Read the model definition and answer for the solid it produces. Units are mm, in the model's axes. Round coordinates to 2 decimals unless told otherwise and drop trailing zeros. Loops run counter-clockwise (first coordinate to the right, second up) from the corner with the lowest first, then second, coordinate; pieces in that order, holes last. Notation, with made-up numbers: M -23.75,72 L -16.75,72 A30 ccw -16.75,101 Z; hole C 28.25,42 d11. An arc over 180 degrees is marked long. Answer as CSV lines item,"result".
Autodesk Inventor part; units mm, degrees
ref_plane "YZ Plane" through (0, 0, 0) normal (1, 0, 0) x (0, 1, 0)
ref_plane "XZ Plane" through (0, 0, 0) normal (0, 1, 0) x (-1, 0, 0)
ref_plane "XY Plane" through (0, 0, 0) normal (0, 0, 1) x (1, 0, 0)
sketch "Sketch1" plane through (0, 0, 0) normal (0, 0, 1) x (1, 0, 0)
  circle A0 centre (0, 0) radius 15.875
  arc A1 (-3.0359, 9.528) -> (-6.5275, 7.5757) centre (0, 0) ccw
  line L0 (0, 0) -> (-5, 8.6603) construction
  line L1 (0, 0) -> (-10.16, 0) construction
  line L2 (-2.058, 7.8342) -> (-3.0359, 9.528)
  line L3 (-5.5564, 5.8937) -> (-6.5275, 7.5757)
  arc A2 (-2.058, 7.8342) -> (-5.5564, 5.8937) centre (0, 0) ccw
  circle A3 centre (0, 0) radius 8.1
  arc A4 (6.7336, 7.3932) -> (3.297, 9.4409) centre (0, 0) ccw
  line L4 (5.7556, 5.6994) -> (6.7336, 7.3932)
  line L5 (2.3259, 7.7589) -> (3.297, 9.4409)
  arc A5 (9.7695, -2.1348) -> (9.8245, 1.8652) centre (0, 0) ccw
  line L6 (7.8136, -2.1348) -> (9.7695, -2.1348)
  line L7 (7.8823, 1.8652) -> (9.8245, 1.8652)
  arc A6 (3.0359, -9.528) -> (6.5275, -7.5757) centre (0, 0) ccw
  line L8 (2.058, -7.8342) -> (3.0359, -9.528)
  line L9 (5.5564, -5.8937) -> (6.5275, -7.5757)
  arc A7 (-6.7336, -7.3932) -> (-3.297, -9.4409) centre (0, 0) ccw
  line L10 (-5.7556, -5.6994) -> (-6.7336, -7.3932)
  line L11 (-2.3259, -7.7589) -> (-3.297, -9.4409)
  arc A8 (-9.7695, 2.1348) -> (-9.8245, -1.8652) centre (0, 0) ccw
  line L12 (-7.8136, 2.1348) -> (-9.7695, 2.1348)
  line L13 (-7.8823, -1.8652) -> (-9.8245, -1.8652)
  point P0 (5, 8.6603)
  point P1 (10, 0)
  point P2 (5, -8.6603)
  point P3 (-5, -8.6603)
  point P4 (-10, 0)
  dimension "d5" = 16.2
  dimension "d0" = 31.75
  dimension "d2" = 60
  dimension "d3" = 4
  dimension "d4" = 20
  dimension "d8" = 360
extrude "Extrusion1" add sketch "Sketch1" along normal blind 25.4 contours A0 | L2 A2 L3 A1 | A3 A2 | L5 A4 L4 A3 | A3 L13 A8 L12 | L7 A5 L6 A3 | A3 L11 A7 L10 | A3 L9 A6 L8
extrude "Extrusion2" cut sketch "Sketch1" along normal blind 15.24 contours A3 A2
extrude "Extrusion3" cut sketch "Sketch1" along normal blind 15.24 contours L2 A2 L3 A1
pattern_circular "Circular Pattern1" count 6 over 360 about axis through (0, 0, 0) along (0, 0, 1) of "Extrusion3"
sketch "Sketch2" plane through (0, 0, 15.24) normal (0, 0, -1) x (-1, 0, 0)
  arc A0 (9.8245, -1.8652) -> (9.7695, 2.1348) centre (0, 0) ccw
  circle A1 centre (0, 0) radius 4.7625
  dimension "d19" = 9.525
extrude "Extrusion4" cut sketch "Sketch2" against normal blind 7.62
sketch "Sketch4" plane through (0, 0, 0) normal (1, 0, 0) x (0, 1, 0)
  line L0 (8.1, 0) -> (8.1, 15.24)
  line L1 (8.1, 15.24) -> (4.7625, 15.24)
  line L2 (4.7625, 15.24) -> (4.7625, 22.86)
  line L3 (4.7625, 22.86) -> (-4.7625, 22.86)
  line L4 (-4.7625, 22.86) -> (-4.7625, 15.24)
  line L5 (-4.7625, 15.24) -> (-8.1, 15.24)
  line L6 (-8.1, 15.24) -> (-8.1, 0)
  line L7 (-8.1, 0) -> (-15.875, 0)
  line L8 (-15.875, 0) -> (-15.875, 25.4)
  line L9 (-15.875, 25.4) -> (15.875, 25.4)
  line L10 (15.875, 25.4) -> (15.875, 0)
  line L11 (15.875, 0) -> (8.1, 0)
  line L12 (0, 25.4) -> (0, 50.8)
  line L13 (0, 50.8) -> (-6.35, 50.8)
  line L14 (-6.35, 50.8) -> (-6.35, 38.1)
  line L15 (-6.35, 38.1) -> (-15.875, 25.4)
  point P0 (0, 0)
  dimension "d22" = 25.4
  dimension "d23" = 6.35
  dimension "d24" = 12.7
revolve "Revolution1" add sketch "Sketch4" angle 360 about axis through (0, 0, 25.4) along (0, 0, 1) contours L9 L15 L14 L13 L12
sketch "Sketch5" plane through (0, 0, 0) normal (0, 1, 0) x (-1, 0, 0)
  line L0 (10, 0) -> (10, 15.24)
  line L1 (10, 15.24) -> (4.7625, 15.24)
  line L2 (4.7625, 15.24) -> (4.7625, 22.86)
  line L3 (4.7625, 22.86) -> (-4.7625, 22.86)
  line L4 (-4.7625, 22.86) -> (-4.7625, 15.24)
  line L5 (-4.7625, 15.24) -> (-10, 15.24)
  line L6 (-10, 15.24) -> (-10, 0)
  line L7 (-10, 0) -> (-15.875, 0)
  line L8 (-15.875, 0) -> (-15.875, 25.4)
  line L9 (-15.875, 25.4) -> (-6.35, 38.1)
  line L10 (-6.35, 38.1) -> (-6.35, 50.8)
  line L11 (-6.35, 50.8) -> (6.35, 50.8)
  line L12 (6.35, 50.8) -> (6.35, 38.1)
  line L13 (6.35, 38.1) -> (15.875, 25.4)
  line L14 (15.875, 25.4) -> (15.875, 0)
  line L15 (15.875, 0) -> (10, 0)
  point P0 (0, 0)
  dimension "d26" = 25.4
  dimension "d27" = 12.7
properties part number "motor connector"
1) Straight lines are drawn through the part: line 1 (Y direction, x = 0, z = 18) (1 decimal); line 2 (Z direction, x = -5.5, y = -1); line 3 (Y direction, x = 3, z = 21.5). For each, find the intervals that lie inside material, in ascending order.
Evaluation:
line 1,"y = -15.9 to -4.8, 4.8 to 15.9"
line 2,"z = 15.24 to 50.8"
line 3,"y = -15.59 to -3.7, 3.7 to 15.59"
2) Each of these flat-tipped pins is pushed along its axis until it touches: P1, Ø1, axis at x = 4.5, y = -7.5, coming from the +Z side; P2, Ø5.5, axis at x = -3, y = 1, coming from the -Z side; P3, Ø1.6, axis at x = -8.5, z = 7, coming from the -Y side. Where does it stop, or does it pass through?
Evaluation:
P1,"stops at z = 35.57"
P2,"stops at z = 15.24"
P3,"stops at y = -13.88"
3) Determine the mould class of faces 1 (the cylindrical face through (6.2, 1.38, 44.36)), 2 (the flat face through (7, -7, 0)), 3 (the flat face through (6.238, 6.534, 7.513)) for opening direction X: released by +X, released by -X, zero draft, split by the parting line, or undercut.
Evaluation:
face 1,"split by the parting line"
face 2,"zero draft"
face 3,"undercut"
4) Find section D-D, the plane z = 42. Give the vertices of the cut face in (x, y), then the cut area to 3 significant figures.
Evaluation:
outline,"C 0,0 d12.7"
area,"127 mm^2"
